```python
from build123d import *

# Parameters (mm, degrees)
SKETCH_R     = 6.75
PAD_DEPTH    = 25
SKETCH001_R  = 15
PAD001_DEPTH = 3
CHAMFER_SIZE = 3


with BuildPart() as part:
    # Sketch → Pad (new body)
    with BuildSketch(Plane.XY):
        Circle(SKETCH_R)
    extrude(amount=PAD_DEPTH)

    # Sketch001 → Pad001 (join)
    with BuildSketch(Plane.XY):
        Circle(SKETCH001_R)
    extrude(amount=PAD001_DEPTH)

    # Chamfer
    chamfer_edges = [part.edges().sort_by_distance(p)[0] for p in [
        (-6.75, 0, 25),
    ]]
    chamfer(chamfer_edges, length=CHAMFER_SIZE)


solid = part.part
```
The listing builds one solid part. Answer for the finished solid, in the listing's coordinates (mm). A direction names the side the tool comes from. Round coordinates to 2 decimals unless told otherwise and drop trailing zeros. Loops run counter-clockwise (first coordinate to the right, second up) from the corner with the lowest first, then second, coordinate; pieces in that order, holes last. Notation, with made-up numbers: (38, 6) - (49, 6) arc R27 cw to (49, 24) - close; hole circle Ø10 at (12.5, 66.5). An arc over 180 degrees is marked (long way). Return JSON: item names as keys, results as strings. Group by question number.
1. Each of these flat-tipped pins is pushed along its axis until it touches: P1, Ø2, axis at y = -2.5, z = 16, coming from the +X side; P2, Ø1, axis at x = 6, z = 8.5, coming from the +Y side; P3, Ø10, axis at x = -11.5, y = 8.5, coming from the +Z side. Where does it stop, or does it pass through?
2. The part is cut by section A-A on x = 0. Determine the outline of the cut face in (y, z), then the cut area to 3 significant figures.
3. The part is cut by section D-D on z = 2.25. Determine the outline of the cut face in (x, y).
4. The part is cut by section C-C on z = 20. Determine the outline of the cut face in (x, y), then the cut area to 3 significant figures.
5. Which of the six approach directions +Z, -Z, +X, -X, +Y, -Y give full straight-line access (tool end or side, diameter ignored) to faces 1 (the flat face through (0, 0, 25)), 2 (the flat face through (3.1, -6.5, 3))?
6. Consider probe 1 along Z at (x, y) = (-9.5, 3.5); probe 2 along X at (y, z) = (0, 4.25); probe 3 along X at (y, z) = (4.75, 4.5). Determine where each line is inside the solid, lowest interval first.
Resolved:
{
 "1": {"P1": "stops at x = 6.58", "P2": "stops at y = 3.91", "P3": "stops at z = 3"},
 "2": {"outline": "(-15, 0) - (15, 0) - (15, 3) - (6.75, 3) - (6.75, 22) - (3.75, 25) - (-3.75, 25) - (-6.75, 22) - (-6.75, 3) - (-15, 3) - close", "area": "378 mm²"},
 "3": {"outline": "circle Ø30 at (0, 0)"},
 "4": {"outline": "circle Ø13.5 at (0, 0)", "area": "143 mm²"},
 "5": {"face 1": "+Z, +X, -X, +Y, -Y", "face 2": "+Z"},
 "6": {"probe 1": "z = 0 to 3", "probe 2": "x = -6.75 to 6.75", "probe 3": "x = -4.8 to 4.8"}
}
